```python
from build123d import *

# Parameters (mm, degrees)
F0_R      = 26
F0_R_2    = 22.5
F1_DEPTH  = 20
F2_R      = 23.5
F2_R_2    = 22.5
F3_DEPTH  = 5
F4_R      = 23.5
F4_R_2    = 22.5
F5_DEPTH  = 5
F7_DEPTH  = 2
F9_DEPTH  = 5
F11_DEPTH = 2
F12_R     = 22.5
F12_R_2   = 22
F13_DEPTH = 6
F14_R     = 23
F14_R_2   = 22.5
F15_DEPTH = 2


with BuildPart() as f1:
    # F0 (on Top) → F1 (new body)
    with BuildSketch(Plane.XY):
        Circle(F0_R)
        Circle(F0_R_2, mode=Mode.SUBTRACT)
    extrude(amount=F1_DEPTH)

    # F2 (on face) → F3 (cut)
    with BuildSketch(Plane(origin=(0, 0, 0), x_dir=(1, 0, 0), z_dir=(0, 0, -1))):
        Circle(F2_R)
        Circle(F2_R_2, mode=Mode.SUBTRACT)
    extrude(amount=-F3_DEPTH, mode=Mode.SUBTRACT)

    # F4 (on face) → F5 (join)
    with BuildSketch(Plane.XY.offset(20)):
        Circle(F4_R)
        Circle(F4_R_2, mode=Mode.SUBTRACT)
    extrude(amount=F5_DEPTH)

    # F6 (on face) → F7 (join)
    with BuildSketch(Plane.XY.offset(25)):
        with BuildLine():
            Line((-20.3515969889, 11.75), (-20.7846096908, 12))
            ThreePointArc((-20.7846096908, 12), (-24, 0), (-20.7846096908, -12))
            Line((-20.7846096908, -12), (-20.3515969889, -11.75))
            ThreePointArc((-20.3515969889, -11.75), (-23.5, 0), (-20.3515969889, 11.75))
        make_face()
        with BuildLine():
            Line((20.3515969889, 11.75), (20.7846096908, 12))
            ThreePointArc((20.7846096908, 12), (12, 20.7846096908), (0, 24))
            Line((0, 24), (0, 23.5))
            ThreePointArc((0, 23.5), (11.75, 20.3515969889), (20.3515969889, 11.75))
        make_face()
        with BuildLine():
            ThreePointArc((0, -24), (12, -20.7846096908), (20.7846096908, -12))
            Line((20.7846096908, -12), (20.3515969889, -11.75))
            ThreePointArc((20.3515969889, -11.75), (11.75, -20.3515969889), (0, -23.5))
            Line((0, -23.5), (0, -24))
        make_face()
    extrude(amount=-F7_DEPTH)

    # F8 (on face) → F9 (cut)
    with BuildSketch(Plane(origin=(0, 0, 0), x_dir=(1, 0, 0), z_dir=(0, 0, -1))):
        with BuildLine():
            Line((20.3515969889, 11.75), (20.7846096908, 12))
            ThreePointArc((20.7846096908, 12), (12, 20.7846096908), (0, 24))
            Line((0, 24), (0, 23.5))
            ThreePointArc((0, 23.5), (11.75, 20.3515969889), (20.3515969889, 11.75))
        make_face()
        with BuildLine():
            ThreePointArc((0, -24), (12, -20.7846096908), (20.7846096908, -12))
            Line((20.7846096908, -12), (20.3515969889, -11.75))
            ThreePointArc((20.3515969889, -11.75), (11.75, -20.3515969889), (0, -23.5))
            Line((0, -23.5), (0, -24))
        make_face()
        with BuildLine():
            Line((-20.3515969889, 11.75), (-20.7846096908, 12))
            ThreePointArc((-20.7846096908, 12), (-24, 0), (-20.7846096908, -12))
            Line((-20.7846096908, -12), (-20.3515969889, -11.75))
            ThreePointArc((-20.3515969889, -11.75), (-23.5, 0), (-20.3515969889, 11.75))
        make_face()
    extrude(amount=-F9_DEPTH, mode=Mode.SUBTRACT)

    # F10 (on face) → F11 (cut)
    with BuildSketch(Plane(origin=(0, 0, 5), x_dir=(1, 0, 0), z_dir=(0, 0, -1))):
        with BuildLine():
            ThreePointArc((20.3515969889, 11.75), (22.6992569178, 6.0822475599), (23.5, 0))
            ThreePointArc((23.5, 0), (22.6992569178, -6.0822475599), (20.3515969889, -11.75))
            Line((20.3515969889, -11.75), (20.7846096908, -12))
            ThreePointArc((20.7846096908, -12), (23.1822198309, -6.2116570825), (24, 0))
            ThreePointArc((24, 0), (23.1822198309, 6.2116570825), (20.7846096908, 12))
            Line((20.7846096908, 12), (20.3515969889, 11.75))
        make_face()
        with BuildLine():
            Line((0, -24), (0, -23.5))
            ThreePointArc((0, -23.5), (-11.75, -20.3515969889), (-20.3515969889, -11.75))
            Line((-20.3515969889, -11.75), (-20.7846096908, -12))
            ThreePointArc((-20.7846096908, -12), (-12, -20.7846096908), (0, -24))
        make_face()
        with BuildLine():
            ThreePointArc((-20.3515969889, 11.75), (-11.75, 20.3515969889), (0, 23.5))
            Line((0, 23.5), (0, 24))
            ThreePointArc((0, 24), (-12, 20.7846096908), (-20.7846096908, 12))
            Line((-20.7846096908, 12), (-20.3515969889, 11.75))
        make_face()
    extrude(amount=F11_DEPTH, mode=Mode.SUBTRACT)

    # F12 (on face) → F13 (join)
    with BuildSketch(Plane(origin=(0, 0, 5), x_dir=(1, 0, 0), z_dir=(0, 0, -1))):
        Circle(F12_R)
        Circle(F12_R_2, mode=Mode.SUBTRACT)
    extrude(amount=-F13_DEPTH)

    # F14 (on face) → F15 (cut)
    with BuildSketch(Plane.XY.offset(11)):
        Circle(F14_R)
        Circle(F14_R_2, mode=Mode.SUBTRACT)
    extrude(amount=F15_DEPTH, mode=Mode.SUBTRACT)


solid = f1.part
```
Design review of the part built by this model. Coordinates are the model's own, in mm. A direction names the side the tool comes from. Coordinates: 2 decimals unless noted, no trailing zeros. Order: outer loops, then holes, each group sorted by start corner. A loop starts at its lowest first (then second) coordinate and runs counter-clockwise, first axis right, second up. Notation, with made-up numbers: (-17, 55) -> (33, 55) arc R31 ccw to (33, 92) -> close; hole circle Ø11 at (-9, 37). An arc over 180 degrees is marked (long way). One line per item, written item: value. Start each with the question number.
Q1. For probe 1 along Y at (x, z) = (0, 11.8); probe 2 along Z at (x, y) = (22.5, 2.5); probe 3 along Y at (x, z) = (0, 22), list the stretches that pass through material, from the lowest coordinate up.
Q2. Take a section at A-A, the plane y = -20. State the section outline as (x, z) points.
Q3. Tool access review of faces 1 (the flat face through (11.9, -20.6, 23)), 2 (the flat face through (-12, -20.6, 3)), 3 (the cylindrical face through (10.382, -19.961, 18.916)), 4 (the cylindrical face through (-24, 0, 24)), 5 (the cylindrical face through (12.152, 20.696, 24.014)): name each direction out of +Z, -Z, +X, -X, +Y, -Y from which nothing blocks a thin tool from reaching the whole face with its end or side.
Q4. Insertion check: pin 1 Ø24 at (x, y) = (-2, 2) entering from -Z; pin 2 Ø1.5 at (x, z) = (-7, 7.5) entering from +Y; pin 3 Ø3 at (x, y) = (-21.5, 5) entering from -Z; pin 4 Ø4 at (y, z) = (-10.5, 3) entering from -X. Each pin has a flat end and moves straight along its axis. Give the tip position at first contact, or say it passes through.
Q5. Take a section at C-C, the plane z = 21. State the section outline as (x, y) points, then the cut area to 3 significant figures.
Q6. Mouldability with a two-part tool opening along Z and no side actions: class faces 6 (the flat face through (23, -6, 0)), 7 (the flat face through (-23.7, 0.1, 23)), 8 (the flat face through (23, 0, 25)) as pulls with the +Z half, pulls with the -Z half, needs draft (parallel to the pull), parting line crosses it, or undercut.
Q7. Take a section at D-D, the plane z = 17.5. State the section outline as (x, y) points.
Q8. Take a section at B-B, the plane x = 5. State the section outline as (y, z) points.
Values follow:
1. probe 1: y = -26 to -23, 23 to 26
1. probe 2: z = 5 to 11, 13 to 25
1. probe 3: y = -23.5 to -22.5, 22.5 to 23.5
2. outline: (-16.61, 0) -> (-12.34, 0) -> (-12.34, 3) -> (-13.27, 3) -> (-13.27, 5) -> (-9.17, 5) -> (-9.17, 11) -> (-11.36, 11) -> (-11.36, 13) -> (-10.31, 13) -> (-10.31, 25) -> (-12.34, 25) -> (-12.34, 20) -> (-16.61, 20) -> close; (9.17, 5) -> (13.27, 5) -> (13.27, 0) -> (16.61, 0) -> (16.61, 20) -> (12.34, 20) -> (12.34, 23) -> (13.27, 23) -> (13.27, 25) -> (10.31, 25) -> (10.31, 13) -> (11.36, 13) -> (11.36, 11) -> (9.17, 11) -> close
3. face 1: +X, -Y
3. face 2: none
3. face 3: +Z
3. face 4: +Z, -X
3. face 5: +Z, +X, +Y
4. pin 1: passes through
4. pin 2: stops at y = 25.24
4. pin 3: stops at z = 5
4. pin 4: stops at x = -24.57
5. outline: circle Ø47 at (0, 0); hole circle Ø45 at (0, 0)
5. area: 145 mm2
6. face 6: pulls with the -Z half
6. face 7: undercut
6. face 8: pulls with the +Z half
7. outline: circle Ø52 at (0, 0); hole circle Ø45 at (0, 0)
8. outline: (-25.51, 0) -> (-23.47, 0) -> (-23.47, 5) -> (-21.42, 5) -> (-21.42, 11) -> (-22.45, 11) -> (-22.45, 13) -> (-21.94, 13) -> (-21.94, 25) -> (-23.47, 25) -> (-23.47, 23) -> (-22.96, 23) -> (-22.96, 20) -> (-25.51, 20) -> close; (21.42, 5) -> (23.47, 5) -> (23.47, 0) -> (25.51, 0) -> (25.51, 20) -> (22.96, 20) -> (22.96, 23) -> (23.47, 23) -> (23.47, 25) -> (21.94, 25) -> (21.94, 13) -> (22.45, 13) -> (22.45, 11) -> (21.42, 11) -> close
